```python
from build123d import *

# Parameters (mm, degrees)
SKETCH1_W           = 65
SKETCH1_H           = 47
SKETCH1_R           = 12.25
SKETCH1_R_2         = 1.623849847
BOSS_EXTRUDE1_DEPTH = 3.7
FILLET1_R           = 3


with BuildPart() as part:
    # Sketch1 → Boss-Extrude1 (new body)
    with BuildSketch(Plane(origin=(0, 0, 0), x_dir=(1, 0, 0), z_dir=(0, 1, 0))):
        with Locations((15.646990036, 10.777629745)):
            Rectangle(SKETCH1_W, SKETCH1_H)
        with Locations((4.096990036, 10.777629745)):
            Circle(SKETCH1_R, mode=Mode.SUBTRACT)
        with Locations((-11.403009964, -4.722370255)):
            Circle(SKETCH1_R_2, mode=Mode.SUBTRACT)
        with Locations((18.596990036, -4.722370255)):
            Circle(SKETCH1_R_2, mode=Mode.SUBTRACT)
        with Locations((18.596990036, 25.277629745)):
            Circle(SKETCH1_R_2, mode=Mode.SUBTRACT)
        with Locations((-11.403009964, 25.277629745)):
            Circle(SKETCH1_R_2, mode=Mode.SUBTRACT)
        with BuildLine():
            Line((39.356990036, 0.777629745), (40.336990036, 0.777629745))
            ThreePointArc((40.336990036, 0.777629745), (42.746990036, -1.632370255), (40.336990036, -4.042370255))
            Line((40.336990036, -4.042370255), (39.356990036, -4.042370255))
            ThreePointArc((39.356990036, -4.042370255), (36.946990036, -1.632370255), (39.356990036, 0.777629745))
        make_face(mode=Mode.SUBTRACT)
        with BuildLine():
            Line((39.356990036, 20.777629745), (40.336990036, 20.777629745))
            ThreePointArc((40.336990036, 20.777629745), (42.746990036, 23.187629745), (40.336990036, 25.597629745))
            Line((40.336990036, 25.597629745), (39.356990036, 25.597629745))
            ThreePointArc((39.356990036, 25.597629745), (36.946990036, 23.187629745), (39.356990036, 20.777629745))
        make_face(mode=Mode.SUBTRACT)
    extrude(amount=BOSS_EXTRUDE1_DEPTH)

    # Fillet1
    fillet1_edges = [part.edges().sort_by_distance(p)[0] for p in [
        (-16.853009964, 1.85, -34.277629745),
        (48.146990036, 1.85, -34.277629745),
        (48.146990036, 1.85, 12.722370255),
        (-16.853009964, 1.85, 12.722370255),
    ]]
    fillet(fillet1_edges, radius=FILLET1_R)


solid = part.part
```
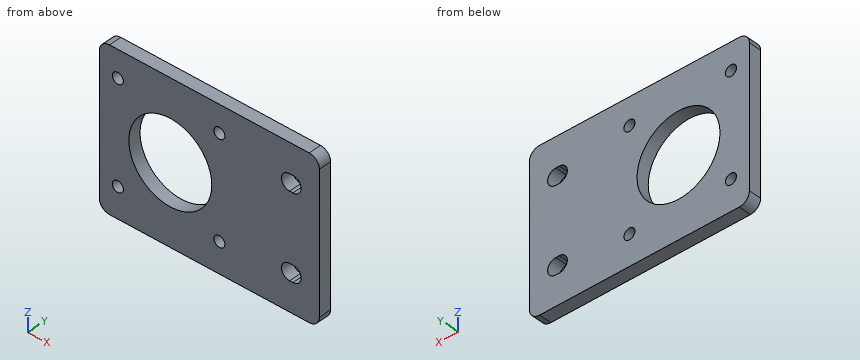
Check sheet for the modelled part. Datum: model origin and axes. Units: mm. Round coordinates to 2 decimals unless told otherwise and drop trailing zeros. Loops run counter-clockwise (first coordinate to the right, second up) from the corner with the lowest first, then second, coordinate; pieces in that order, holes last. Notation, with made-up numbers: (59.25, 14) - (92.25, 14) arc R23 cw to (92.25, 35) - close; hole circle Ø10 at (-36, 73). An arc over 180 degrees is marked (long way). Write item = value, one per line. Start each with the question number.
Q1. Section check B-B (z = -12.5). Record the boundary of the cut face in (x, y).
Q2. Section check A-A (x = 10.5). Record the boundary of the cut face in (y, z), plus the area to 3 significant figures.
Q3. Section check C-C (y = 0.8). Record the boundary of the cut face in (x, z), plus the area to 3 significant figures.
Q4. Thickness scan on L1, parallel to Z at x = -11.5, y = 1.95; L2, parallel to Z at x = -3, y = 2.75; L3, parallel to Z at x = 11, y = 3.15. Record the ranges inside material, lowest first.
Derived:
q1.outline = (-16.85, 0) - (-8.03, 0) - (-8.03, 3.7) - (-16.85, 3.7) - close; (16.23, 0) - (48.15, 0) - (48.15, 3.7) - (16.23, 3.7) - close
q2.outline = (0, -34.28) - (3.7, -34.28) - (3.7, -21.22) - (0, -21.22) - close; (0, -0.33) - (3.7, -0.33) - (3.7, 12.72) - (0, 12.72) - close
q2.area = 96.6 mm^2
q3.outline = (-16.85, -31.28) arc R3 ccw to (-13.85, -34.28) - (45.15, -34.28) arc R3 ccw to (48.15, -31.28) - (48.15, 9.72) arc R3 ccw to (45.15, 12.72) - (-13.85, 12.72) arc R3 ccw to (-16.85, 9.72) - close; hole circle Ø3.25 at (-11.4, -25.28); hole circle Ø3.25 at (-11.4, 4.72); hole circle Ø24.5 at (4.1, -10.78); hole circle Ø3.25 at (18.6, -25.28); hole circle Ø3.25 at (18.6, 4.72); hole (39.36, -25.6) - (40.34, -25.6) arc R2.41 ccw to (40.34, -20.78) - (39.36, -20.78) arc R2.41 ccw to start; hole (39.36, -0.78) - (40.34, -0.78) arc R2.41 ccw to (40.34, 4.04) - (39.36, 4.04) arc R2.41 ccw to start
q3.area = 2,500 mm^2
q4.L1 = -34.28 to -26.9, -23.66 to 3.1, 6.34 to 12.72
q4.L2 = -34.28 to -20.76, -0.79 to 12.72
q4.L3 = -34.28 to -20.9, -0.66 to 12.72
